Can you work these out from the model? Positions are in its coordinate system, mm. A direction names the side the tool comes from. Coordinates: 2 decimals unless noted, no trailing zeros. Order: outer loops, then holes, each group sorted by start corner. A loop starts at its lowest first (then second) coordinate and runs counter-clockwise, first axis right, second up. Notation, with made-up numbers: (56, 57) -> (96, 57) arc R20 cw to (96, 77) -> close; hole circle Ø7 at (46, 68). An arc over 180 degrees is marked (long way). Write item = value, one per line.
```python
from build123d import *

# Parameters (mm, degrees)
F0_R     = 7.5
F1_DEPTH = 20
F2_R     = 1.190625
F3_DEPTH = 76.94342
F5_R     = 7.5
F6_DEPTH = 15
F7_SIZE  = 6


with BuildPart() as f1:
    # F0 (on Top) → F1 (new body)
    with BuildSketch(Plane.XY):
        Circle(F0_R)
    extrude(amount=-F1_DEPTH)

    # F2 (on Top) → F3 (join, symmetric)
    with BuildSketch(Plane.XY):
        Circle(F2_R)
    extrude(amount=F3_DEPTH, both=True)

    # F5 (on offset) → F6 (join)
    with BuildSketch(Plane.XY.offset(25)):
        Circle(F5_R)
    extrude(amount=F6_DEPTH)

    # F7
    f7_edges = [f1.edges().sort_by_distance(p)[0] for p in [
        (-7.5, 0, 40),
    ]]
    chamfer(f7_edges, length=F7_SIZE)


solid = f1.part
```
Item 1: If we mould it in two halves opening along Z, with no side actions, what happens to faces 4 (the flat face through (2, 0, -20)), 5 (the flat face through (2, 0, 0)), 6 (the cylindrical face through (-0.945, -0.724, -48.073))? For each: pulls with the +Z half, pulls with the -Z half, needs draft (parallel to the pull), parting line crosses it, or undercut.
A:
face_4 = pulls with the -Z half
face_5 = undercut
face_6 = needs draft
Item 2: For faces 1 (the cylindrical face through (-0.945, -0.724, 12.675)), 2 (the flat face through (0, 0, 76.943)), 3 (the cylindrical face through (-0.945, -0.724, 58.73)), which set-ups out of +Z, -Z, +X, -X, +Y, -Y let a thin tool reach every point of the face, with its end or its side?
A:
face_1 = none
face_2 = +Z, +X, -X, +Y, -Y
face_3 = +Z
Item 3: I want a section at B-B, the plane z = -39.5. Please give me the cut outline in (x, y).
A:
outline = circle Ø2.38 at (0, 0)
Item 4: I want a section at A-A, the plane z = 30.5. Please give me the cut outline in (x, y), plus the area to 3 significant figures.
A:
outline = circle Ø15 at (0, 0)
area = 177 mm2
Item 5: If I drill on probe 1 along Z at (x, y) = (-1, -3.75); probe 2 along Z at (x, y) = (-2, -6.25); probe 3 along Y at (x, z) = (1, -36), over which ranges is the centre line in solid material (lowest first)?
A:
probe_1 = -20 to 0, 25 to 37.62
probe_2 = -20 to 0, 25 to 34.94
probe_3 = -0.65 to 0.65
Item 6: I'm going to push flat-ended pins straight in: P1, Ø5, axis at y = -1.5, z = 40, coming from the -X side; P2, Ø1.5, axis at x = 5.5, z = -17, coming from the -Y side; P3, Ø1, axis at x = -5, y = -3.5, coming from the +Z side. Where does each tip first touch, or does it pass through?
A:
P1 = -3.82
P2 = -5.8
P3 = 35.9
